from build123d import *

# Parameters (mm, degrees)
CYLINDER012_R                      = 1.95
CYLINDER012_DEPTH                  = 10
CYLINDER011_R                      = 1.95
CYLINDER011_DEPTH                  = 10
CYLINDER007_R                      = 2.525
CYLINDER007_DEPTH                  = 37
CYLINDER008_R                      = 4.75
CYLINDER008_DEPTH                  = 13
CYLINDER006_R                      = 2.65
CYLINDER006_DEPTH                  = 2
CYLINDER005_R                      = 6.55
CYLINDER005_DEPTH                  = 5
BOX023_W                           = 12
BOX023_H                           = 8
BOX023_DEPTH                       = 10
BOX019_W                           = 2
BOX019_H                           = 6
BOX019_DEPTH                       = 5.9
BOX020_W                           = 2
BOX020_H                           = 6
BOX020_DEPTH                       = 5.9
CHAMFER004013007011015006006_SIZE  = 1
CYLINDER009_R                      = 2.525
CYLINDER009_DEPTH                  = 10
BOX018_W                           = 20
BOX018_H                           = 20
BOX018_DEPTH                       = 5
FILLET_R                           = 3
BOX021_W                           = 6
BOX021_H                           = 7
BOX021_DEPTH                       = 1
BOX022_W                           = 6
BOX022_H                           = 7
BOX022_DEPTH                       = 1
BOX017_W                           = 31
BOX017_H                           = 20
BOX017_DEPTH                       = 25
CHAMFER004013007011015006005_SIZE2 = 15
CHAMFER004013007011015006005_SIZE  = 17
CHAMFER004013007011015006007_SIZE  = 1
CHAMFER004013007011015006008_SIZE  = 0.4


with BuildPart() as cylinder012:
    # Cylinder012 → Cylinder012 (new body)
    with BuildSketch(Plane(origin=(24, 14, 41), x_dir=(1, 0, 0), z_dir=(0, -1, 0))):
        Circle(CYLINDER012_R)
    extrude(amount=CYLINDER012_DEPTH)


with BuildPart() as fusion004023:
    # Cylinder011 → Cylinder011 (new body)
    with BuildSketch(Plane(origin=(24, -4, 41), x_dir=(1, 0, 0), z_dir=(0, -1, 0))):
        Circle(CYLINDER011_R)
    extrude(amount=CYLINDER011_DEPTH)

    # Fusion004023: union Cylinder012
    add(cylinder012.part)


with BuildPart() as cylinder007:
    # Cylinder007 → Cylinder007 (new body)
    with BuildSketch(Plane(origin=(14, 0, 50), x_dir=(0, 0, -1), z_dir=(1, 0, 0))):
        Circle(CYLINDER007_R)
    extrude(amount=CYLINDER007_DEPTH)


with BuildPart() as fusion004019:
    # Cylinder008 → Cylinder008 (new body)
    with BuildSketch(Plane(origin=(14, 0, 50), x_dir=(0, 0, -1), z_dir=(1, 0, 0))):
        Circle(CYLINDER008_R)
    extrude(amount=CYLINDER008_DEPTH)

    # Fusion004019: union Cylinder007
    add(cylinder007.part)


with BuildPart() as cylinder006:
    # Cylinder006 → Cylinder006 (new body)
    with BuildSketch(Plane.XY.offset(3)):
        Circle(CYLINDER006_R)
    extrude(amount=CYLINDER006_DEPTH)


with BuildPart() as cut028006004005005:
    # Cylinder005 → Cylinder005 (new body)
    with BuildSketch(Plane.XY):
        Circle(CYLINDER005_R)
    extrude(amount=CYLINDER005_DEPTH)

    # Cut028006004005005: cut Cylinder006
    add(cylinder006.part, mode=Mode.SUBTRACT)


with BuildPart() as cut028006004005005_1:
    # Cut028006004005005 placement: moved
    add(cut028006004005005.part.moved(Location((22, 0, 33))))


with BuildPart() as fusion004022:
    # Box023 → Box023 (new body)
    with BuildSketch(Plane(origin=(7, -4, 28), x_dir=(1, 0, 0), z_dir=(0, 0, 1))):
        with Locations((6, 4)):
            Rectangle(BOX023_W, BOX023_H)
    extrude(amount=BOX023_DEPTH)

    # Fusion004022: union Cut028006004005005
    add(cut028006004005005_1.part)


with BuildPart() as cube019:
    # Box019 → Box019 (new body)
    with BuildSketch(Plane(origin=(46, -10, 47), x_dir=(1, 0, 0), z_dir=(0, 0, 1))):
        with Locations((1, 3)):
            Rectangle(BOX019_W, BOX019_H)
    extrude(amount=BOX019_DEPTH)


with BuildPart() as chamfer004013007011015006006:
    # Box020 → Box020 (new body)
    with BuildSketch(Plane(origin=(46, 4, 47), x_dir=(1, 0, 0), z_dir=(0, 0, 1))):
        with Locations((1, 3)):
            Rectangle(BOX020_W, BOX020_H)
    extrude(amount=BOX020_DEPTH)

    # Fusion004018: union Cube019
    add(cube019.part)

    # Chamfer004013007011015006006
    chamfer004013007011015006006_edges = [chamfer004013007011015006006.edges().sort_by_distance(p)[0] for p in [
        (48, 7, 47),
        (48, -7, 47),
    ]]
    chamfer(chamfer004013007011015006006_edges, length=CHAMFER004013007011015006006_SIZE)


with BuildPart() as cylinder009:
    # Cylinder009 → Cylinder009 (new body)
    with BuildSketch(Plane(origin=(57, 0, 32), x_dir=(1, 0, 0), z_dir=(0, 0, 1))):
        Circle(CYLINDER009_R)
    extrude(amount=CYLINDER009_DEPTH)


with BuildPart() as fillet_body:
    # Box018 → Box018 (new body)
    with BuildSketch(Plane(origin=(47, -10, 35), x_dir=(1, 0, 0), z_dir=(0, 0, 1))):
        with Locations((10, 10)):
            Rectangle(BOX018_W, BOX018_H)
    extrude(amount=BOX018_DEPTH)

    # Fillet
    fillet_edges = [fillet_body.edges().sort_by_distance(p)[0] for p in [
        (67, -10, 37.5),
        (67, 10, 37.5),
    ]]
    fillet(fillet_edges, radius=FILLET_R)


with BuildPart() as cube021:
    # Box021 → Box021 (new body)
    with BuildSketch(Plane(origin=(54, -10, 40), x_dir=(1, 0, 0), z_dir=(0, 0, 1))):
        with Locations((3, 3.5)):
            Rectangle(BOX021_W, BOX021_H)
    extrude(amount=BOX021_DEPTH)


with BuildPart() as cut028006004005004:
    # Box022 → Box022 (new body)
    with BuildSketch(Plane(origin=(54, 3, 40), x_dir=(1, 0, 0), z_dir=(0, 0, 1))):
        with Locations((3, 3.5)):
            Rectangle(BOX022_W, BOX022_H)
    extrude(amount=BOX022_DEPTH)

    # Fusion004020: union Fillet body, Cube021
    add(fillet_body.part)
    add(cube021.part)

    # Cut028006004005004: cut Cylinder009
    add(cylinder009.part, mode=Mode.SUBTRACT)


with BuildPart() as obj1:
    # Box017 → Box017 (new body)
    with BuildSketch(Plane(origin=(16, -10, 35), x_dir=(1, 0, 0), z_dir=(0, 0, 1))):
        with Locations((15.5, 10)):
            Rectangle(BOX017_W, BOX017_H)
    extrude(amount=BOX017_DEPTH)

    # Chamfer004013007011015006005
    chamfer004013007011015006005_edges = [obj1.edges().sort_by_distance(p)[0] for p in [
        (16, 0, 60),
    ]]
    chamfer004013007011015006005_side = obj1.faces().sort_by_distance((16, 0, 47.5))[0]
    chamfer(chamfer004013007011015006005_edges, length=CHAMFER004013007011015006005_SIZE, length2=CHAMFER004013007011015006005_SIZE2, reference=chamfer004013007011015006005_side)

    # Fusion004021: union Chamfer004013007011015006006, Cut028006004005004
    add(chamfer004013007011015006006.part)
    add(cut028006004005004.part)

    # Cut028006004005006: cut Fusion004022
    add(fusion004022.part, mode=Mode.SUBTRACT)

    # Chamfer004013007011015006007
    chamfer004013007011015006007_edges = [obj1.edges().sort_by_distance(p)[0] for p in [
        (16, 7, 35),
        (16, -7, 35),
    ]]
    chamfer(chamfer004013007011015006007_edges, length=CHAMFER004013007011015006007_SIZE)

    # Cut028006004005007: cut Fusion004019
    add(fusion004019.part, mode=Mode.SUBTRACT)

    # Chamfer004013007011015006008
    chamfer004013007011015006008_edges = [obj1.edges().sort_by_distance(p)[0] for p in [
        (16, 10, 39.5),
        (16, 0, 43),
        (16, -10, 39.5),
        (16.5, 10, 35.5),
        (23.5, 10, 51.5),
        (32, 10, 35),
        (39, 10, 60),
        (23.5, -10, 51.5),
        (31, 0, 60),
        (16.5, -10, 35.5),
        (32, -10, 35),
        (39, -10, 60),
        (55.5, 10, 35),
        (55.5, -10, 35),
        (66.12132, 9.12132, 35),
        (67, 0, 35),
        (66.12132, -9.12132, 35),
    ]]
    chamfer(chamfer004013007011015006008_edges, length=CHAMFER004013007011015006008_SIZE)

    # Cut028006004005008: cut Fusion004023
    add(fusion004023.part, mode=Mode.SUBTRACT)


solid = obj1.part
Verification items for the finished model (mm, model axes). A direction names the side the tool comes from. Give positions to 0.01 mm unless a question says otherwise; leave off trailing zeros. Order: outer loops, then holes, each group sorted by start corner. A loop starts at its lowest first (then second) coordinate and runs counter-clockwise, first axis right, second up. Notation, with made-up numbers: M -2.75,33 L 44.25,33 A7 ccw 44.25,44 Z; hole C 76,19.5 d3. An arc over 180 degrees is marked long. Answer as a JSON object with one key per item and string values. Group by question number.
1) Access from +Z, -Z, +X, -X, +Y, -Y to the whole of each face (thin tool, end or side, straight path). Record for faces 1 (the face through (24, 4, 41)), 2 (the face through (28.546, -0.228, 36.479)), 3 (the face through (47.5, 7, 52.9)).
2) Cross-section at D-D (y = 5.75). Enter the section's corners in (x, z).
3) Mould release check, pull along Y, two halves, no side actions. Record for faces 4 (the face through (24, -4, 41)), 5 (the face through (23.43, 1.43, 45.47)), 6 (the face through (23.551, 9.803, 51.251)): released by +Y, released by -Y, zero draft, split by the parting line, or undercut.
4) Cross-section at B-B (z = 51). Enter the section's corners in (x, y), then the cut area to 3 significant figures.
5) Cross-section at A-A (x = 41.5). Enter the section's corners in (y, z) (3 decimals), then the cut area to 3 significant figures.
6) Cross-section at C-C (x = 57). Enter the section's corners in (y, z) (3 decimals).
7) Depth check by flat-ended pin: pin 1 Ø1.2 at (x, z) = (25, 41) entering from -Y; pin 2 Ø1.5 at (y, z) = (2.5, 53) entering from +X; pin 3 Ø1 at (y, z) = (7.5, 44.5) entering from -X. Enter the tip coordinate at first touch or a pass-through.
8) Scan lines: line 1 along Z through (x, y) = (31.5, -0.25); line 2 along X through (y, z) = (0, 38.8) (3 decimals); line 3 along Z through (x, y) = (64, -4.5). Record each from-to range of solid material in increasing order. Write a range as [from, to].
Result sheet:
{
 "1": {"face 1": "+Y", "face 2": "-Z", "face 3": "+Z, +X, +Y, -Y"},
 "2": {"outline": "M 16,36 L 17,35 L 18.86,35 L 18.86,38 L 25.14,38 L 25.14,35 L 66.6,35 L 67,35.4 L 67,40 L 60,40 L 60,41 L 54,41 L 54,40 L 47,40 L 47,47 L 48,48 L 48,52.9 L 47,52.9 L 47,60 L 31.4,60 L 30.74,59.7 L 16.26,43.3 L 16,42.6 Z; hole C 24,41 d3.9"},
 "3": {"face 4": "released by -Y", "face 5": "undercut", "face 6": "released by +Y"},
 "4": {"outline": "M 23.06,-9.6 L 23.59,-10 L 48,-10 L 48,-4 L 47,-4 L 47,-2.32 L 27,-2.32 L 27,-4.64 L 23.06,-4.64 Z; M 23.06,4.64 L 27,4.64 L 27,2.32 L 47,2.32 L 47,4 L 48,4 L 48,10 L 23.59,10 L 23.06,9.6 Z", "area": "361 mm2"},
 "5": {"outline": "M -10,35.4 L -9.6,35 L 9.6,35 L 10,35.4 L 10,59.6 L 9.6,60 L -9.6,60 L -10,59.6 Z; hole C 0,50 d5.05", "area": "480 mm2"},
 "6": {"outline": "M -10,35.4 L -9.6,35 L -2.525,35 L -2.525,40 L -3,40 L -3,41 L -10,41 Z; M 2.525,35 L 9.6,35 L 10,35.4 L 10,41 L 3,41 L 3,40 L 2.525,40 Z"},
 "7": {"pin 1": "stops at y = -4", "pin 2": "stops at x = 47", "pin 3": "stops at x = 16.88"},
 "8": {"line 1": "z = [35, 47.49], [52.51, 60]", "line 2": "x = [16, 54.475], [59.525, 67]", "line 3": "z = [35, 40]"}
}
